from build123d import *

# Parameters (mm, degrees)
SKETCH_1_R          = 2.1
EXTRUDE_1_DEPTH     = 3
SKETCH_2_R          = 2.1
SKETCH_2_R_2        = 1.6
CUT_EXTRUDE_1_DEPTH = 3
FILLET_1_R          = 3
SKETCH_5_R          = 1.55
CUT_EXTRUDE_3_DEPTH = 10
CUT_EXTRUDE_4_DEPTH = 3
FILLET_5_R          = 1.5


with BuildPart() as part:
    # 草图1 → 凸台-拉伸1 (new body)
    with BuildSketch(Plane(origin=(0, 0, 0), x_dir=(1, 0, 0), z_dir=(0, 1, 0))):
        with BuildLine():
            Line((-22.5, 0), (-22.5, 35))
            Line((-22.5, 35), (22.5, 35))
            Line((22.5, 35), (22.5, 0))
            ThreePointArc((22.5, 0), (21.870970759, -17.545046315), (19.98711306, -35))
            Line((19.98711306, -35), (-25.586313325, -35))
            ThreePointArc((-25.586313325, -35), (-23.273072434, -17.56790632), (-22.5, 0))
        make_face()
        with Locations(Location((0, 0, 0), (0, 0, 270))):
            Circle(SKETCH_1_R, mode=Mode.SUBTRACT)
    extrude(amount=EXTRUDE_1_DEPTH)

    # 草图2 → 切除-拉伸1 (cut)
    with BuildSketch(Plane(origin=(0, 3, 0), x_dir=(1, 0, 0), z_dir=(0, 1, 0))):
        with Locations(Location((-16.51288694, -28, 0), (0, 0, 270))):
            Circle(SKETCH_2_R)
        with Locations(Location((8.48711306, -28, 0), (0, 0, 270))):
            Circle(SKETCH_2_R)
        with Locations(Location((-12.5, 29, 0), (0, 0, 270))):
            Circle(SKETCH_2_R_2)
        with Locations(Location((12.5, 29, 0), (0, 0, 270))):
            Circle(SKETCH_2_R_2)
    extrude(amount=-CUT_EXTRUDE_1_DEPTH, mode=Mode.SUBTRACT)

    # 圆角1
    fillet_1_edges = [part.edges().sort_by_distance(p)[0] for p in [
        (-22.5, 1.5, -35),
        (22.5, 1.5, -35),
        (19.98711306, 1.5, 35),
        (-25.586313325, 1.5, 35),
    ]]
    fillet(fillet_1_edges, radius=FILLET_1_R)

    # 草图5 → 切除-拉伸3 (cut)
    with BuildSketch(Plane.XZ):
        with Locations(Location((14.5, 0, 0), (0, 0, 270))):
            Circle(SKETCH_5_R)
        with Locations(Location((14.5, -20, 0), (0, 0, 270))):
            Circle(SKETCH_5_R)
    extrude(amount=-CUT_EXTRUDE_3_DEPTH, mode=Mode.SUBTRACT)

    # 草图6 → 切除-拉伸4 (cut)
    with BuildSketch(Plane(origin=(0, 3, 0), x_dir=(1, 0, 0), z_dir=(0, 1, 0))):
        Polygon((7.439955283, 22.5), (-12.439955283, 22.5), (-2.5, 16.039029066), align=None)
        Polygon((-5.25235241, 14.25), (-16, 21.235970934), (-16, 7.264029066), align=None)
        Polygon((7.439955283, 6), (-2.5, 12.460970934), (-12.439955283, 6), align=None)
        Polygon((11, 21.235970934), (0.25235241, 14.25), (11, 7.264029066), align=None)
        Polygon((7.646201615, -6), (-12.646201615, -6), (-2.5, -12.93323777), align=None)
        Polygon((-5.158676434, -14.75), (-16, -7.34176223), (-16, -22.15823777), align=None)
        Polygon((7.646201615, -23.5), (-2.5, -16.56676223), (-12.646201615, -23.5), align=None)
        Polygon((11, -7.34176223), (0.158676434, -14.75), (11, -22.15823777), align=None)
    extrude(amount=-CUT_EXTRUDE_4_DEPTH, mode=Mode.SUBTRACT)

    # 圆角5
    fillet_5_edges = [part.edges().sort_by_distance(p)[0] for p in [
        (-12.646201615, 1.5, 6),
        (7.646201615, 1.5, 6),
        (11, 1.5, -21.235970934),
        (11, 1.5, -7.264029066),
        (0.25235241, 1.5, -14.25),
        (-5.25235241, 1.5, -14.25),
        (-16, 1.5, -7.264029066),
        (-16, 1.5, -21.235970934),
        (-2.5, 1.5, -12.460970934),
        (7.439955283, 1.5, -6),
        (-12.439955283, 1.5, -6),
        (11, 1.5, 7.34176223),
        (11, 1.5, 22.15823777),
        (0.158676434, 1.5, 14.75),
        (-16, 1.5, 7.34176223),
        (-5.158676434, 1.5, 14.75),
        (-16, 1.5, 22.15823777),
        (-2.5, 1.5, 16.56676223),
        (7.646201615, 1.5, 23.5),
        (-12.646201615, 1.5, 23.5),
        (-12.439955283, 1.5, -22.5),
        (7.439955283, 1.5, -22.5),
        (-2.5, 1.5, -16.039029066),
    ]]
    fillet(fillet_5_edges, radius=FILLET_5_R)


solid = part.part
The listing builds one solid part. Answer for the finished solid, in the listing's coordinates (mm). A direction names the side the tool comes from. Give positions to 0.01 mm unless a question says otherwise; leave off trailing zeros. Write each loop counter-clockwise with the first axis right and the second up, starting at its lowest first coordinate (ties: lowest second). Pieces come first, ordered by that corner, then holes. Notation, with made-up numbers: (-31, -20) - (5, -20) arc R9 ccw to (5, -10) - close; hole circle Ø9 at (-31.5, -35). An arc over 180 degrees is marked (long way). One line per question, with ' | ' between items. Start each with the question number.
1. Section A-A, the plane x = 0 is taken. Determine the outline of the cut face in (y, z), then the cut area to 3 significant figures.
2. Straight lines are drawn through the part: line 1 (X direction, y = 0.4, z = -15.5); line 2 (X direction, y = 1.4, z = -29); line 3 (X direction, y = 0.7, z = 11). For each, find the intervals that lie inside material, in ascending order.
3. For faces 1 (the face through (0.526, 1.521, 10.865)), 2 (the face through (22.5, 1, -16)), determine the directions among +Z, -Z, +X, -X, +Y, -Y from which every point of the face is accessible in a straight line to the end or side of a thin tool.
4. Section B-B, the plane y = 1.7 is taken. Count the separate pieces of the cut face and the enclosed holes in it, then the cut area to 3 significant figures.
5. Determine the mould class of faces 3 (the face through (-9.217, 1.479, 22.468)), 4 (the face through (21.977, 1.479, 16.007)), 5 (the face through (0, 1, -35)), 6 (the face through (-23.144, 1.479, 16.034)) for opening direction X: +X half, -X half, draft (parallel to the pull), parting line (faces both ways), or undercut.
6. Given P1, Ø0.9, axis at y = 1.5, z = 13.5, coming from the -X side; P2, Ø1.9, axis at x = 12.5, z = -29, coming from the +Y side; P3, Ø0.9, axis at y = 1.5, z = 13, coming from the +X side; P4, Ø0.9, axis at y = 2, z = -13, coming from the -X side, each flat-ended and moving along its own axis, determine where each tip first touches the part or whether it passes through.
7. Section C-C, the plane z = 25 is taken. Determine the outline of the cut face in (x, y).
Result:
1) outline: (0, -35) - (3, -35) - (3, -22.5) - (0, -22.5) - close; (0, -17.66) - (3, -17.66) - (3, -10.84) - (0, -10.84) - close; (0, -6) - (3, -6) - (3, -2.1) - (0, -2.1) - close; (0, 2.1) - (3, 2.1) - (3, 6) - (0, 6) - close; (0, 11.22) - (3, 11.22) - (3, 18.28) - (0, 18.28) - close; (0, 23.5) - (3, 23.5) - (3, 35) - (0, 35) - close | area: 137 mm2
2) line 1: x = -22.5 to -16, -7.18 to 2.18, 11 to 22.5 | line 2: x = -22.5 to -14.1, -10.9 to 10.9, 14.1 to 22.5 | line 3: x = -22.8 to -16, -10.65 to -5.33, 0.33 to 5.65, 11 to 22.25
3) face 1: +Y, -Y | face 2: +Z, -Z, +X, +Y, -Y
4) separate pieces: 1 | enclosed holes: 15 | area: 2,550 mm2
5) face 3: undercut | face 4: +X half | face 5: draft | face 6: -X half
6) P1: stops at x = -22.99 | P2: passes through | P3: stops at x = 22.18 | P4: stops at x = -22.5
7) outline: (-24.07, 0) - (21.22, 0) - (21.22, 3) - (-24.07, 3) - close
